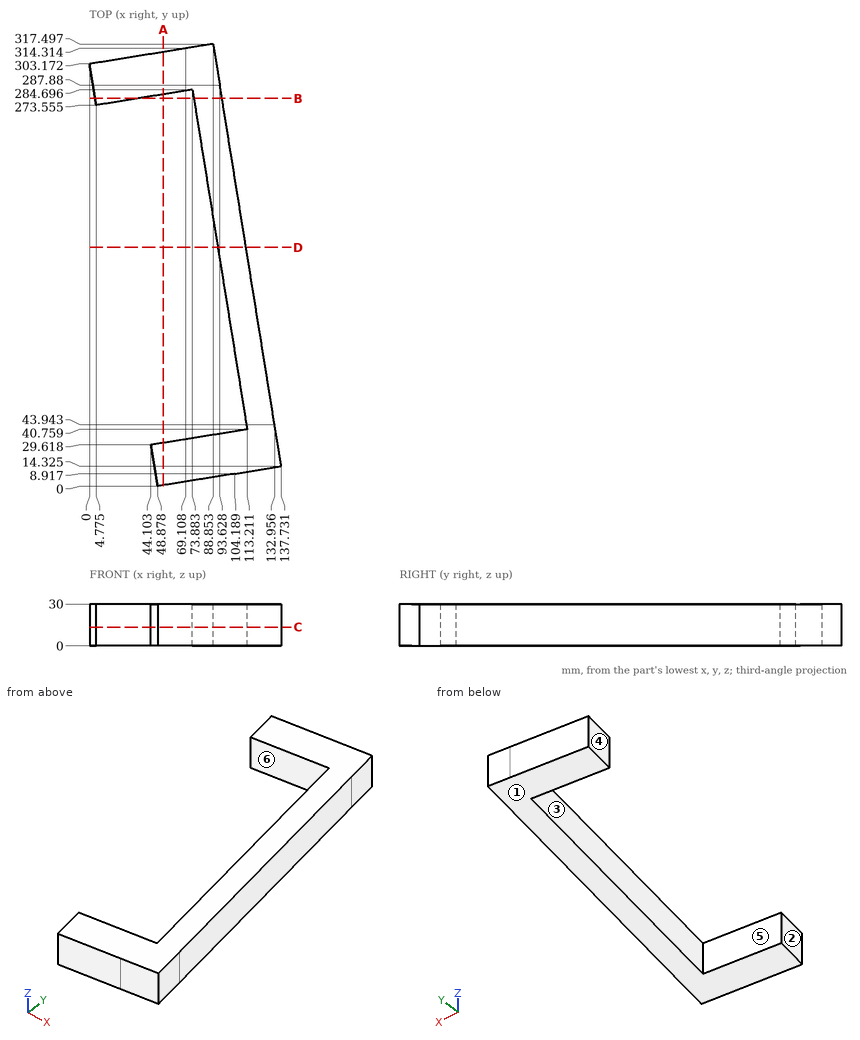
Print and shaded views of the part. All mm, measured from the part's lowest x, y and z. A direction names the side the tool comes from. Coordinates: 2 decimals unless noted, no trailing zeros. Write each loop counter-clockwise with the first axis right and the second up, starting at its lowest first coordinate (ties: lowest second). Pieces come first, ordered by that corner, then holes. Notation, with made-up numbers: M 60,67 L 118,67 A20 ccw 118,71 Z; hole C 32,8 d1. An arc over 180 degrees is marked long. Return JSON: item names as keys, results as strings.
1. Probe L1, parallel to Y at x = 57, z = 19.5 (1 decimal); L2, parallel to Y at x = 73, z = 24.25 (1 decimal); L3, parallel to X at y = 181.5, z = 21.5. List the from-to ranges inside material, lowest first.
Determined:
{"L1": "1.3 to 31.7, 282 to 312.4", "L2": "3.9 to 34.3, 284.6 to 314.9", "L3": "90.52 to 110.78"}
2. 3-axis set-ups, long thin cutter, end or side, ignore diameter. For the marked faces 4, 5 and 6: which of +Z, -Z, +X, -X, +Y, -Y reach the whole face in a straight line?
Determined:
{"face 4": "+Z, -Z, -X, -Y", "face 5": "+Z, -Z, -X", "face 6": "+Z, -Z"}
3. Saw through at B-B, the plane y = 278.5. Write the cut outline in (x, z).
Determined:
{"outline": "M 3.98,0 L 35.45,0 L 35.45,30 L 3.98,30 Z; M 74.88,0 L 95.14,0 L 95.14,30 L 74.88,30 Z"}
4. Saw through at A-A, the plane x = 53. Write the cut outline in (y, z) (1 decimal).
Determined:
{"outline": "M 0.7,0 L 31.1,0 L 31.1,30 L 0.7,30 Z; M 281.3,0 L 311.7,0 L 311.7,30 L 281.3,30 Z"}
5. Saw through at D-D, the plane y = 171.5. Write the cut outline in (x, z).
Determined:
{"outline": "M 92.13,0 L 112.39,0 L 112.39,30 L 92.13,30 Z"}
6. Pull direction Y, two halves, no side cores. Call the marked faces 1, 2 and 3: pulls with the +Y half, pulls with the -Y half, needs draft (parallel to the pull), parting line crosses it, or undercut.
Determined:
{"face 1": "needs draft", "face 2": "pulls with the -Y half", "face 3": "undercut"}
7. Flat gauge pins, fed straight in: pin 1 Ø4 at (x, z) = (81.5, 12.5) entering from +Y (1 decimal); pin 2 Ø8 at (x, y) = (19.5, 279) entering from -Z; pin 3 Ø8 at (y, z) = (171, 4) entering from +X; pin 4 Ø5 at (x, z) = (54, 10.5) entering from +Y. Where does each tip first touch, or does it go through?
Determined:
{"pin 1": "y = 316.6", "pin 2": "z = 0", "pin 3": "x = 113.12", "pin 4": "y = 312.28"}
8. Saw through at C-C, the plane z = 13.5. Write the cut outline in (x, y) (1 decimal).
Determined:
{"outline": "M 0,303.2 L 4.8,273.6 L 73.9,284.7 L 113.2,40.8 L 44.1,29.6 L 48.9,0 L 104.2,8.9 L 137.7,14.3 L 88.9,317.5 L 69.1,314.3 Z"}
